from build123d import *

# Parameters (mm, degrees)
ESBO_O1_W                = 110
ESBO_O1_H                = 70
RESSALTO_EXTRUS_O1_DEPTH = 2
ESBO_O2_W                = 70
ESBO_O2_H                = 110
RESSALTO_EXTRUS_O2_DEPTH = 2
ESBO_O3_W                = 70
ESBO_O3_H                = 110
RESSALTO_EXTRUS_O3_DEPTH = 2
ESBO_O4_R                = 7.5
CORTE_EXTRUS_O1_DEPTH    = 6.35
ESBO_O5_R                = 2.5
CORTE_EXTRUS_O2_DEPTH    = 10
ESBO_O6_R                = 2.5
CORTE_EXTRUS_O3_DEPTH    = 10
ESBO_O7_R                = 13.5
ESBO_O7_R_2              = 1
CORTE_EXTRUS_O5_DEPTH    = 10
ESBO_O9_R                = 5
CORTE_EXTRUS_O6_DEPTH    = 160.452187191
ESBO_O10_R               = 2.5
CORTE_EXTRUS_O7_DEPTH    = 2
CORTE_EXTRUS_O11_REACH   = 128.151
ESBO_O18_R               = 2.5
ESBO_O19_R               = 1.5
CORTE_EXTRUS_O12_DEPTH   = 10
CORTE_EXTRUS_O13_REACH   = 161.452


with BuildPart() as part:
    # Esboço1 → Ressalto-extrusão1 (new body)
    with BuildSketch(Plane(origin=(0, 0, 0), x_dir=(1, 0, 0), z_dir=(0, 1, 0))):
        Rectangle(ESBO_O1_W, ESBO_O1_H)
    extrude(amount=RESSALTO_EXTRUS_O1_DEPTH)

    # Esboço2 → Ressalto-extrusão2 (add)
    with BuildSketch(Plane.ZY.offset(55)):
        with Locations((0, 55)):
            Rectangle(ESBO_O2_W, ESBO_O2_H)
    extrude(amount=-RESSALTO_EXTRUS_O2_DEPTH)

    # Esboço3 → Ressalto-extrusão3 (add)
    with BuildSketch(Plane(origin=(55, 0, 0), x_dir=(0, 0, -1), z_dir=(1, 0, 0))):
        with Locations((0, 55)):
            Rectangle(ESBO_O3_W, ESBO_O3_H)
    extrude(amount=-RESSALTO_EXTRUS_O3_DEPTH)

    # Esboço4 → Corte-extrusão1 (cut)
    with BuildSketch(Plane(origin=(0, 2, 0), x_dir=(1, 0, 0), z_dir=(0, 1, 0))):
        with Locations(Location((-17, 0, 0), (0, 0, 270))):
            Circle(ESBO_O4_R)
    extrude(amount=-CORTE_EXTRUS_O1_DEPTH, mode=Mode.SUBTRACT)

    # Esboço5 → Corte-extrusão2 (cut)
    with BuildSketch(Plane(origin=(55, 0, 0), x_dir=(0, 0, -1), z_dir=(1, 0, 0))):
        with Locations((-7, 10)):
            Circle(ESBO_O5_R)
    extrude(amount=-CORTE_EXTRUS_O2_DEPTH, mode=Mode.SUBTRACT)

    # Esboço6 → Corte-extrusão3 (cut)
    with BuildSketch(Plane(origin=(55, 0, 0), x_dir=(0, 0, -1), z_dir=(1, 0, 0))):
        with Locations((-18.3, 98.5)):
            Circle(ESBO_O6_R)
        with Locations((26.3, 47.5)):
            Circle(ESBO_O6_R)
    extrude(amount=-CORTE_EXTRUS_O3_DEPTH, mode=Mode.SUBTRACT)

    # Esboço7 → Corte-extrusão5 (cut)
    with BuildSketch(Plane.ZY.offset(-53)):
        with Locations((18.3, 53.5)):
            Circle(ESBO_O7_R)
        with Locations((18.3, 53.5)):
            Circle(ESBO_O7_R_2, mode=Mode.SUBTRACT)
        with Locations((18.3, 53.5)):
            Circle(ESBO_O7_R_2)
    extrude(amount=-CORTE_EXTRUS_O5_DEPTH, mode=Mode.SUBTRACT)

    # Esboço9 → Corte-extrusão6 (cut, through all)
    with BuildSketch(Plane(origin=(55, 0, 0), x_dir=(0, 0, -1), z_dir=(1, 0, 0))):
        with Locations((14.2, 53.5)):
            Circle(ESBO_O9_R)
    extrude(amount=-CORTE_EXTRUS_O6_DEPTH, mode=Mode.SUBTRACT)

    # Esboço10 → Corte-extrusão7 (cut)
    with BuildSketch(Plane(origin=(55, 0, 0), x_dir=(0, 0, -1), z_dir=(1, 0, 0))):
        with Locations((25.5, 11.5)):
            Circle(ESBO_O10_R)
        with Locations((25.5, 100.5)):
            Circle(ESBO_O10_R)
    extrude(amount=-CORTE_EXTRUS_O7_DEPTH, mode=Mode.SUBTRACT)

    # Esboço18 → Corte-extrusão11 (cut, up to next)
    with BuildSketch(Plane(origin=(0, 2, 0), x_dir=(1, 0, 0), z_dir=(0, 1, 0)), mode=Mode.PRIVATE) as corte_extrus_o11_sk1:
        with Locations(Location((29, 25, 0), (0, 0, 270))):
            Circle(ESBO_O18_R)
    corte_extrus_o11_tool1 = extrude(corte_extrus_o11_sk1.sketch, amount=-CORTE_EXTRUS_O11_REACH, mode=Mode.PRIVATE) & part.part
    # Esboço18 → Corte-extrusão11 (cut, up to next)
    with BuildSketch(Plane(origin=(0, 2, 0), x_dir=(1, 0, 0), z_dir=(0, 1, 0)), mode=Mode.PRIVATE) as corte_extrus_o11_sk2:
        with Locations(Location((29, -25, 0), (0, 0, 270))):
            Circle(ESBO_O18_R)
    corte_extrus_o11_tool2 = extrude(corte_extrus_o11_sk2.sketch, amount=-CORTE_EXTRUS_O11_REACH, mode=Mode.PRIVATE) & part.part
    add(corte_extrus_o11_tool1.solids().sort_by_distance((29, 2, -25))[0], mode=Mode.SUBTRACT)
    add(corte_extrus_o11_tool2.solids().sort_by_distance((29, 2, 25))[0], mode=Mode.SUBTRACT)

    # Esboço19 → Corte-extrusão12 (cut)
    with BuildSketch(Plane(origin=(0, 2, 0), x_dir=(1, 0, 0), z_dir=(0, 1, 0))):
        with Locations(Location((-17, 13.75, 0), (0, 0, 270))):
            Circle(ESBO_O19_R)
        with Locations(Location((-17, -13.75, 0), (0, 0, 270))):
            Circle(ESBO_O19_R)
    extrude(amount=-CORTE_EXTRUS_O12_DEPTH, mode=Mode.SUBTRACT)

    # Esboço20 → Corte-extrusão13 (cut, up to next)
    with BuildSketch(Plane.ZY.offset(55), mode=Mode.PRIVATE) as corte_extrus_o13_sk1:
        with BuildLine():
            ThreePointArc((-17.7, 31), (-14.2, 27.5), (-10.7, 31))
            ThreePointArc((-10.7, 31), (-14.2, 34.5), (-17.7, 31))
        make_face()
    corte_extrus_o13_tool1 = extrude(corte_extrus_o13_sk1.sketch, amount=-CORTE_EXTRUS_O13_REACH, mode=Mode.PRIVATE) & part.part
    # Esboço20 → Corte-extrusão13 (cut, up to next)
    with BuildSketch(Plane.ZY.offset(55), mode=Mode.PRIVATE) as corte_extrus_o13_sk2:
        with BuildLine():
            ThreePointArc((-17.7, 76), (-14.2, 72.5), (-10.7, 76))
            ThreePointArc((-10.7, 76), (-14.2, 79.5), (-17.7, 76))
        make_face()
    corte_extrus_o13_tool2 = extrude(corte_extrus_o13_sk2.sketch, amount=-CORTE_EXTRUS_O13_REACH, mode=Mode.PRIVATE) & part.part
    add(corte_extrus_o13_tool1.solids().sort_by_distance((-55, 31, -14.2))[0], mode=Mode.SUBTRACT)
    add(corte_extrus_o13_tool2.solids().sort_by_distance((-55, 76, -14.2))[0], mode=Mode.SUBTRACT)


solid = part.part
Read the model definition and answer for the solid it produces. Units are mm, in the model's axes. A direction names the side the tool comes from. Give positions to 0.01 mm unless a question says otherwise; leave off trailing zeros. Write each loop counter-clockwise with the first axis right and the second up, starting at its lowest first coordinate (ties: lowest second). Pieces come first, ordered by that corner, then holes. Notation, with made-up numbers: (28.5, 40.25) - (73.5, 40.25) arc R19 cw to (73.5, 76.25) - close; hole circle Ø9 at (84.25, 83.25). An arc over 180 degrees is marked (long way). Use CSV: the item, a comma, the result in double quotes. Start each with the question number.
Item 1: The mould has two halves that part along Z. Classify faces 1 (the flat face through (-24.7, 1.8, -35)), 2 (the flat face through (-24.7, 1.8, 35)), 3 (the flat face through (-1, 2, 0)), 4 (the cylindrical face through (54.014, 56.879, -10.515)): pulls with the +Z half, pulls with the -Z half, needs draft (parallel to the pull), parting line crosses it, or undercut.
Item 2: Flat-ended cylindrical pins translate along their axes: P1, Ø1.5, axis at x = -0.5, z = 15, coming from the +Y side; P2, Ø5.5, axis at y = 31, z = -14.2, coming from the -X side. Find the tip coordinate at first contact, or state that the pin passes through.
Item 3: The part is cut by section C-C, the plane z = -0.5. Give the vertices of the cut face in (x, y).
Item 4: Consider line 1 (Y direction, x = 53.5, z = 18.3); line 2 (Y direction, x = -53.6, z = -14.2); line 3 (X direction, y = 15, z = -11). Determine where each line is inside the solid, lowest interval first.
Item 5: The part is cut by section A-A, the plane y = 53.5. Give the vertices of the cut face in (x, z), and give its area (3 significant figures).
Item 6: For faces 5 (the flat face through (-53, 57, 0)), 6 (the cylindrical face through (-54.014, 72.583, -14.959)), 7 (the flat face through (55, 54, 0)), 8 (the cylindrical face through (54.01, 102.98, -25.17)), 9 (the flat face through (-55, 54, 0)), determine the directions among +Z, -Z, +X, -X, +Y, -Y from which every point of the face is accessible in a straight line to the end or side of a thin tool.
Item 7: The part is cut by section B-B, the plane y = 26. Give the vertices of the cut face in (x, z), and give its area (3 significant figures).
Item 8: The part is cut by section D-D, the plane z = -26. Give the vertices of the cut face in (x, y).
Taken from the geometry:
1,face 1,"pulls with the -Z half"
1,face 2,"pulls with the +Z half"
1,face 3,"needs draft"
1,face 4,"undercut"
2,P1,"y = 2"
2,P2,"x = 53"
3,outline,"(-55, 0) - (-24.48, 0) - (-24.48, 2) - (-53, 2) - (-53, 110) - (-55, 110) - close; (-9.52, 0) - (55, 0) - (55, 110) - (53, 110) - (53, 2) - (-9.52, 2) - close"
4,line 1,"0 to 40, 67 to 96, 101 to 110"
4,line 2,"0 to 27.5, 34.5 to 48.5, 58.5 to 72.5, 79.5 to 110"
4,line 3,"-55 to -53, 53 to 55"
5,outline,"(-55, -35) - (-53, -35) - (-53, -19.2) - (-55, -19.2) - close; (-55, -9.2) - (-53, -9.2) - (-53, 35) - (-55, 35) - close; (53, -35) - (55, -35) - (55, -19.2) - (53, -19.2) - close; (53, -9.2) - (55, -9.2) - (55, 4.8) - (53, 4.8) - close; (53, 31.8) - (55, 31.8) - (55, 35) - (53, 35) - close"
5,area,"186 mm2"
6,face 5,"+Z, -Z, +Y"
6,face 6,"-X"
6,face 7,"+Z, -Z, +X, +Y, -Y"
6,face 8,"+X"
6,face 9,"+Z, -Z, -X, +Y, -Y"
7,outline,"(-55, -35) - (-53, -35) - (-53, 35) - (-55, 35) - close; (53, -35) - (55, -35) - (55, 35) - (53, 35) - close"
7,area,"280 mm2"
8,outline,"(-55, 0) - (26.71, 0) - (26.71, 2) - (-53, 2) - (-53, 110) - (-55, 110) - close; (31.29, 0) - (55, 0) - (55, 9.05) - (53, 9.05) - (53, 2) - (31.29, 2) - close; (53, 13.95) - (55, 13.95) - (55, 45.02) - (53, 45.02) - close; (53, 49.98) - (55, 49.98) - (55, 98.05) - (53, 98.05) - close; (53, 102.95) - (55, 102.95) - (55, 110) - (53, 110) - close"
